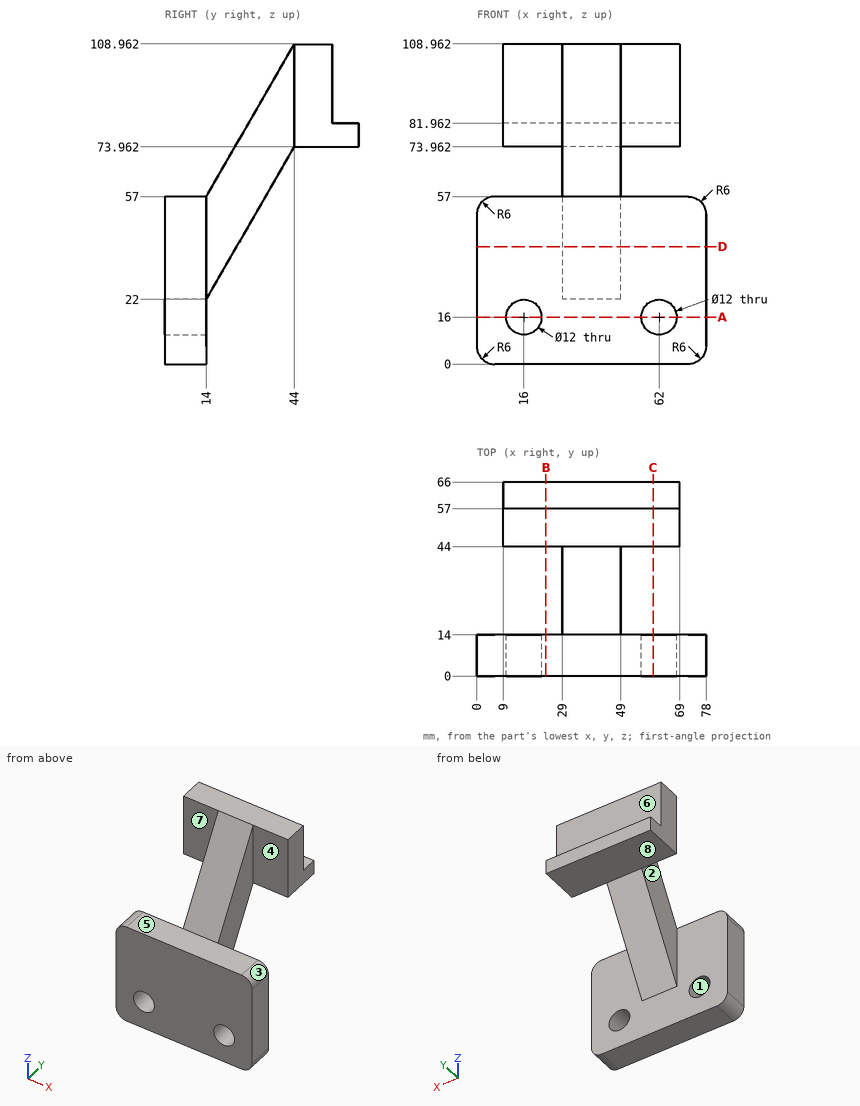
Part print with two shaded views. Sizes in mm from the minimum x, y, z corner. A direction names the side the tool comes from. Coordinates: 2 decimals unless noted, no trailing zeros. Loops run counter-clockwise (first coordinate to the right, second up) from the corner with the lowest first, then second, coordinate; pieces in that order, holes last. Notation, with made-up numbers: (77.25, 76) - (130.25, 76) arc R25 cw to (130.25, 91) - close; hole circle Ø6 at (26.5, -2.5). An arc over 180 degrees is marked (long way). Write each question's results on one line, items separated by ' | '. Start each with the question number.
Q1. Drop flat-ended pins along their axis: pin 1 Ø1.5 at (x, z) = (67.5, 92.5) entering from -Y; pin 2 Ø1.5 at (x, z) = (18.5, 36) entering from +Y; pin 3 Ø24 at (y, z) = (35, 58.5) entering from +X; pin 4 Ø7 at (x, z) = (16, 16) entering from +Y. Give the stop position or say it passes through.
Q2. Two-plate mould, pull along X, no slides. Class the marked faces 1, 2, 3 and 4: +X half, -X half, draft (parallel to the pull), parting line (faces both ways), or undercut.
Q3. Which spindle directions (+Z, -Z, +X, -X, +Y, -Y) get a long thin tool onto all of the face, cutting with end or side? Do the marked faces 5, 6, 7 and 8. Say none if no direction does.
Q4. Slice it at B-B on x = 23.5. Give the cut face in (y, z), and give its area (4 significant figures).
Q5. Slice it at C-C on x = 60. Give the cut face in (y, z), and give its area (3 significant figures).
Q6. Probe line 1 along X through (y, z) = (10.75, 16); line 2 along Y through (x, z) = (68, 32.5); line 3 along X through (y, z) = (31, 65.5). List the from-to ranges inside material, lowest first.
Q7. Slice it at D-D on z = 40. Give the cut face in (x, y).
Q8. Slice it at A-A on z = 16. Give the cut face in (x, y).
Answer:
1) pin 1: stops at y = 44 | pin 2: stops at y = 14 | pin 3: stops at x = 49 | pin 4: passes through
2) face 1: undercut | face 2: -X half | face 3: +X half | face 4: draft
3) face 5: +Z, +X, -X, -Y | face 6: +Z, +X, -X, +Y | face 7: +Z, -Z, -X, -Y | face 8: -Z, +X, -X, +Y
4) outline: (0, 0) - (14, 0) - (14, 57) - (0, 57) - close; (44, 73.96) - (66, 73.96) - (66, 81.96) - (57, 81.96) - (57, 108.96) - (44, 108.96) - close | area: 1,325 mm2
5) outline: (0, 0) - (14, 0) - (14, 10.34) - (0, 10.34) - close; (0, 21.66) - (14, 21.66) - (14, 57) - (0, 57) - close; (44, 73.96) - (66, 73.96) - (66, 81.96) - (57, 81.96) - (57, 108.96) - (44, 108.96) - close | area: 1,170 mm2
6) line 1: x = 0 to 10, 22 to 56, 68 to 78 | line 2: y = 0 to 14 | line 3: x = 29 to 49
7) outline: (0, 0) - (78, 0) - (78, 14) - (49, 14) - (49, 24.39) - (29, 24.39) - (29, 14) - (0, 14) - close
8) outline: (0, 0) - (10, 0) - (10, 14) - (0, 14) - close; (22, 0) - (56, 0) - (56, 14) - (22, 14) - close; (68, 0) - (78, 0) - (78, 14) - (68, 14) - close
